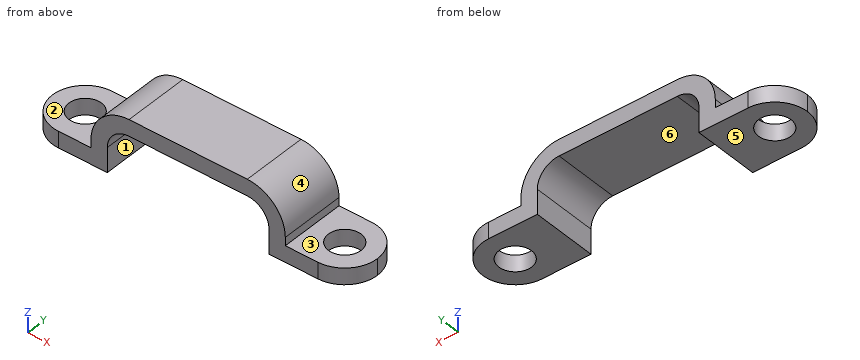
from build123d import *

# Parameters (mm, degrees)
F1_DEPTH = 6
F2_R     = 1.5
F3_DEPTH = 1.5


with BuildPart() as f1:
    # F0 (on Front) → F1 (new body)
    with BuildSketch(Plane.XZ):
        with BuildLine():
            Line((-1.5, 0), (0, 0))
            Line((0, 0), (0, 2.25))
            ThreePointArc((0, 2.25), (0.585786, 3.664214), (2, 4.25))
            Line((2, 4.25), (12.875, 4.25))
            ThreePointArc((12.875, 4.25), (14.289214, 3.664214), (14.875, 2.25))
            Line((14.875, 2.25), (14.875, 0))
            Line((14.875, 0), (16.375, 0))
            Line((16.375, 0), (16.375, 2.25))
            ThreePointArc((16.375, 2.25), (15.349874, 4.724874), (12.875, 5.75))
            Line((12.875, 5.75), (2, 5.75))
            ThreePointArc((2, 5.75), (-0.474874, 4.724874), (-1.5, 2.25))
            Line((-1.5, 2.25), (-1.5, 0))
        make_face()
    extrude(amount=F1_DEPTH)

    # F2 (on Top) → F3 (join)
    with BuildSketch(Plane.XY):
        with BuildLine():
            Line((-1.5, -6), (-1.5, 0))
            Line((-1.5, 0), (-4.5, 0))
            ThreePointArc((-4.5, 0), (-6.62132, -0.87868), (-7.5, -3))
            ThreePointArc((-7.5, -3), (-6.62132, -5.12132), (-4.5, -6))
            Line((-4.5, -6), (-1.5, -6))
        make_face()
        with Locations((-4.5, -3)):
            Circle(F2_R, mode=Mode.SUBTRACT)
        with BuildLine():
            Line((16.375, 0), (16.375, -6))
            Line((16.375, -6), (19.375, -6))
            ThreePointArc((19.375, -6), (21.49632, -5.12132), (22.375, -3))
            ThreePointArc((22.375, -3), (21.49632, -0.87868), (19.375, 0))
            Line((19.375, 0), (16.375, 0))
        make_face()
        with Locations((19.375, -3)):
            Circle(F2_R, mode=Mode.SUBTRACT)
    extrude(amount=F3_DEPTH)


solid = f1.part
CAD build for the part. Positions are in the model's coordinates, mm. Face numbers are marked on the shaded views. A direction names the side the tool comes from. Coordinates: 2 decimals unless noted, no trailing zeros. Write each loop counter-clockwise with the first axis right and the second up, starting at its lowest first coordinate (ties: lowest second). Pieces come first, ordered by that corner, then holes. Notation, with made-up numbers: M 61.5,-25.75 L 96.5,-25.75 A27 ccw 96.5,6.25 Z; hole C 46.5,-2.75 d5. An arc over 180 degrees is marked long. Answer as a JSON object with one key per item and string values. Group by question number.
1) Pin check, flat tips, straight feed: pin 1 Ø1 at (y, z) = (-1.5, 1.5) entering from -X; pin 2 Ø3.5 at (x, y) = (19.375, -3) entering from +Z; pin 3 Ø0.8 at (y, z) = (-4, 2) entering from +X (3 decimals); pin 4 Ø1.5 at (x, z) = (6.5, 2.5) entering from -Y. Stop position of each tip, or through.
2) Tool access for the marked faces 1, 2 and 3: list every direction of +Z, -Z, +X, -X, +Y, -Y with a clear straight run to the whole face (end or side of a thin tool).
3) Wall check: line 1 (X direction, y = -1.5, z = 2.25) (3 decimals); line 2 (Y direction, x = -4.5, z = 1); line 3 (Z direction, x = 5, y = -4.75). Give the ranges that are in metal, low to high. Write a range as from..to.
4) Mould opens along X. For the marked faces 4, 5 and 6 say: +X half, -X half, draft (parallel to the pull), parting line (faces both ways), or undercut.
5) Saw through at B-B (x = 18.75). Write the cut outline in (y, z), plus the area to 3 significant figures.
6) Saw through at C-C (z = 3.05). Write the cut outline in (x, y), plus the area to 3 significant figures.
7) Saw through at D-D (y = -4). Write the cut outline in (x, z) (3 decimals), plus the area to 3 significant figures.
8) Saw through at A-A (z = 0.75). Write the cut outline in (x, y) (3 decimals).
Values follow:
{
 "1": {"pin 1": "stops at x = -7.33", "pin 2": "stops at z = 1.5", "pin 3": "stops at x = 16.375", "pin 4": "passes through"},
 "2": {"face 1": "-Z, +Y, -Y", "face 2": "+Z, -X, +Y, -Y", "face 3": "+Z, +X, +Y, -Y"},
 "3": {"line 1": "x = -1.5..0, 14.875..16.375", "line 2": "y = -6..-4.5, -1.5..0", "line 3": "z = 4.25..5.75"},
 "4": {"face 4": "+X half", "face 5": "draft", "face 6": "undercut"},
 "5": {"outline": "M -6,0 L -4.36,0 L -4.36,1.5 L -6,1.5 Z; M -1.64,0 L 0,0 L 0,1.5 L -1.64,1.5 Z", "area": "4.91 mm2"},
 "6": {"outline": "M -1.41,-6 L 0.17,-6 L 0.17,0 L -1.41,0 Z; M 14.71,-6 L 16.28,-6 L 16.28,0 L 14.71,0 Z", "area": "18.9 mm2"},
 "7": {"outline": "M -7.328,0 L -5.618,0 L -5.618,1.5 L -7.328,1.5 Z; M -3.382,0 L 0,0 L 0,2.25 A2 cw 2,4.25 L 12.875,4.25 A2 cw 14.875,2.25 L 14.875,0 L 18.257,0 L 18.257,1.5 L 16.375,1.5 L 16.375,2.25 A3.5 ccw 12.875,5.75 L 2,5.75 A3.5 ccw -1.5,2.25 L -1.5,1.5 L -3.382,1.5 Z; M 20.493,0 L 22.203,0 L 22.203,1.5 L 20.493,1.5 Z", "area": "46.8 mm2"},
 "8": {"outline": "M -7.5,-3 A3 ccw -4.5,-6 L 0,-6 L 0,0 L -4.5,0 A3 ccw Z; M 14.875,-6 L 19.375,-6 A3 ccw 22.375,-3 A3 ccw 19.375,0 L 14.875,0 Z; hole C -4.5,-3 d3; hole C 19.375,-3 d3"}
}
